Input: part model. Units: mm. Frame: model coordinates. A direction names the side the tool comes from. Round coordinates to 2 decimals unless told otherwise and drop trailing zeros. Loops run counter-clockwise (first coordinate to the right, second up) from the corner with the lowest first, then second, coordinate; pieces in that order, holes last. Notation, with made-up numbers: (70, -6.75) -> (112, -6.75) arc R11 ccw to (112, 1.25) -> close; hole circle Ø2 at (8.25, -25.75). An arc over 180 degrees is marked (long way). Answer in a Markdown table with one row per item. Add a question column.
Q1. Mould query, pull axis X, two halves, no side actions, for faces 5 (the face through (5, 40, -17)), 6 (the face through (-30, 40, -19)), 7 (the face through (11, 40, -19)), 8 (the face through (-10, 40, 0)). Classes: pulls with the +X half, pulls with the -X half, needs draft (parallel to the pull), parting line crosses it, or undercut.
Q2. Pin query (flat end, axial travel): pin 1 (5.5 mm diameter, centred on x = -6.5, y = 35.5, fed in from -Z); pin 2 (5 mm diameter, centred on x = 7, y = 40, fed in from +Z); pin 3 (10 mm diameter, centred on y = 44.5, z = -2.5, fed in from +X). Return the tip coordinate at first contact, or that it passes through.
Q3. Reachability of faces 1 (the face through (-10, 40, 3)), 2 (the face through (-22, 40, -7)), 3 (the face through (3, 40, -7)), 4 (the face through (-19, 40, -10)) from +Z, -Z, +X, -X, +Y, -Y: full face, straight path, thin tool, end or side. Return the list, or none.
Q4. Section A-A, the plane x = -26. Output: boundary loops of the cut face in (y, z), and give its area (3 significant figures).
Q5. Ray query, L1, parallel to X at y = 40, z = -18.55; L2, parallel to Y at x = -26, z = -18; L3, parallel to X at y = 33.5, z = -18.25. Return the intervals inside material, ascending. Write a range as from..to.
Q6. Section D-D, the plane y = 35.5. Output: boundary loops of the cut face in (x, z).
Q7. Section C-C, the plane z = -2.25. Output: boundary loops of the cut face in (x, y).
Q8. Section B-B, the plane y = 40. Output: boundary loops of the cut face in (x, z).
Autodesk Fusion 360 part; units mm, degrees
sketch "Sketch1" plane through (0, 0, 0) normal (1, 0, 0) x (0, 1, 0) in component "Integrated frame"
  circle A0 centre (-46.8244, 18.5) radius 1.5
  circle A1 centre (-9.8244, 18.5) radius 1.5
  circle A2 centre (-46.8244, -18.5) radius 1.5
  circle A3 centre (-9.8244, -18.5) radius 1.5
  line L0 (0, 0) -> (0, 35.4619) construction
  line L1 (60, 100) -> (-60, 100)
  line L2 (-60, 100) -> (-60, -100)
  line L3 (-60, -100) -> (60, -100)
  line L4 (60, -100) -> (60, 100)
  line L5 (60, 100) -> (-60, -100) construction
  line L6 (-60, 100) -> (60, -100) construction
  circle A4 centre (46.8244, 18.5) radius 1.5
  circle A5 centre (46.8244, -18.5) radius 1.5
  circle A6 centre (9.8244, -18.5) radius 1.5
  circle A7 centre (9.8244, 18.5) radius 1.5
  line L7 (-18.5, -45.3481) -> (-21.5, -45.3481)
  line L8 (-21.5, -45.3481) -> (-21.5, -70.3481)
  line L9 (-21.5, -70.3481) -> (-18.5, -70.3481)
  line L10 (-18.5, -70.3481) -> (-18.5, -45.3481)
  line L11 (21.5, -45.3481) -> (21.5, -70.3481)
  line L12 (18.5, -70.3481) -> (18.5, -45.3481)
  line L13 (18.5, -45.3481) -> (21.5, -45.3481)
  line L14 (21.5, -70.3481) -> (18.5, -70.3481)
  circle A8 centre (-43.3091, 82.7998) radius 1.5
  circle A9 centre (-21.3091, 82.7998) radius 1.5
  circle A10 centre (21.3091, 82.7998) radius 1.5
  circle A11 centre (43.3091, 82.7998) radius 1.5
  line L15 (0, 0) -> (33.4715, 0) construction
  circle A12 centre (-43.3091, -82.7998) radius 1.5
  circle A13 centre (-21.3091, -82.7998) radius 1.5
  circle A14 centre (43.3091, -82.7998) radius 1.5
  circle A15 centre (21.3091, -82.7998) radius 1.5
  point P0 (-28.3244, 0)
  dimension "d246" = 3
  dimension "d248" = 18.5
  dimension "d249" = 18.5
  dimension "d252" = 37
  dimension "d253" = -37
  dimension "d261" = 120
  dimension "d262" = 200
  dimension "d264" = 3
  dimension "d265" = 25
  dimension "d266" = 18.5
  dimension "d269" = 3
  dimension "d270" = 3
  dimension "d271" = 22
sketch "Sketch1 (2)" plane through (0, 0, 0) normal (0, 0, 1) x (1, 0, 0) in component "MotorClamp"
  line L0 (0, 50) -> (-19, 50)
  line L1 (-19, 50) -> (-19, 30)
  line L2 (-19, 30) -> (0, 30)
  line L3 (0, 30) -> (0, 50)
  line L4 (-19, 50) -> (-22, 50)
  line L5 (-22, 50) -> (-22, 30)
  line L6 (-22, 30) -> (-19, 30)
  line L7 (-19, 30) -> (-19, 50)
  line L8 (0, 50) -> (3, 50)
  line L9 (3, 50) -> (3, 30)
  line L10 (3, 30) -> (0, 30)
  line L11 (0, 30) -> (0, 50)
  dimension "d272" = 19
  dimension "d273" = 20
  dimension "d274" = 3
  dimension "d275" = 3
extrude "Extrude1" add sketch "Sketch1 (2)" along normal blind 3 in component "MotorClamp"
extrude "Extrude2" add sketch "Sketch1 (2)" against normal blind 17 contours L3 L8 L9 L10 L11 | L1 L4 L5 L6 L7 in component "MotorClamp"
extrude "Extrude3" add 2 faces at (-20, 36.6667, -17) (1, 43.3333, -17) along direction (0, 0, -1) blind 3 in component "MotorClamp"
sketch "Sketch2" plane through (0, 0, -20) normal (0, 0, -1) x (1, 0, 0) in component "MotorClamp"
  line L0 (-19, -50) -> (-19, -30)
  line L1 (-19, -30) -> (-22, -30)
  line L2 (-22, -30) -> (-22, -50)
  line L3 (-22, -50) -> (-19, -50)
  line L4 (-22, -30) -> (-30, -30)
  line L5 (-30, -30) -> (-30, -50)
  line L6 (-30, -50) -> (-22, -50)
  line L7 (-22, -50) -> (-22, -30)
  line L8 (3, -50) -> (11, -50)
  line L9 (11, -50) -> (11, -30)
  line L10 (11, -30) -> (3, -30)
  line L11 (3, -30) -> (3, -50)
  line L12 (-30, -30) -> (-22, -50) construction
  line L13 (-30, -50) -> (-22, -30) construction
  line L14 (3, -30) -> (11, -50) construction
  line L15 (3, -50) -> (11, -30) construction
  circle A0 centre (-26, -40) radius 1.55
  circle A1 centre (7, -40) radius 1.55
  dimension "d282" = 8
  dimension "d283" = 8
  dimension "d284" = 25
  dimension "d285" = 3.1
  dimension "d286" = 3.1
extrude "Extrude4" add sketch "Sketch2" against normal blind 3 contours L2 L4 L5 L6 L7 | L8 L9 L10 L11 in component "MotorClamp"
extrude "Extrude1'" [suppressed] in component "Integrated frame"
sketch "Laser cut sketch" plane through (3, 0, 0) normal (1, 0, 0) x (0, 1, 0) in component "Integrated frame"
  circle A0 centre (-9.8244, -18.5) radius 1.5
  circle A1 centre (-46.8244, -18.5) radius 1.5
  circle A2 centre (-46.8244, 18.5) radius 1.5
  circle A3 centre (-9.8244, 18.5) radius 1.5
  circle A4 centre (46.8244, 18.5) radius 1.5
  circle A5 centre (46.8244, -18.5) radius 1.5
  circle A6 centre (9.8244, -18.5) radius 1.5
  circle A7 centre (9.8244, 18.5) radius 1.5
  line L0 (-18.5, -45.3481) -> (-18.5, -70.3481)
  line L1 (-18.5, -70.3481) -> (-21.5, -70.3481)
  line L2 (-21.5, -70.3481) -> (-21.5, -45.3481)
  line L3 (-21.5, -45.3481) -> (-18.5, -45.3481)
  line L4 (21.5, -45.3481) -> (21.5, -70.3481)
  line L5 (21.5, -70.3481) -> (18.5, -70.3481)
  line L6 (18.5, -70.3481) -> (18.5, -45.3481)
  line L7 (18.5, -45.3481) -> (21.5, -45.3481)
  line L8 (60, -100) -> (60, 100)
  line L9 (60, 100) -> (-60, 100)
  line L10 (-60, 100) -> (-60, -100)
  line L11 (-60, -100) -> (60, -100)
extrude "Extrude2'" [suppressed]
component "Integrated frame" placed x (1, 0, 0) y (0, 1, 0) z (0, 0, 1) at (0, 0, 0)
component "MotorClamp" placed x (1, 0, 0) y (0, 1, 0) z (0, 0, 1) at (0, 0, 0)
equation "partLength = 250 mm"
equation "partWidth = 25 mm"
equation "boltHole = 3 mm"
equation "boltFromEdgesClose = 10 mm"
equation "boltGap = 12 mm"
equation "boltFromEdgesFar = 40 mm"
equation "boltGapFromSide = ( partWidth - boltGap ) / 2"
equation "boltGapDiag = boltGap * sqrt(2)"
equation "d246 = boltHole"
equation "d248 = ( 37 / 2 ) * 1 mm"
equation "d249 = ( 37 / 2 ) * 1 mm"
equation "d266 = ( 37 / 2 ) * 1 mm"
equation "d269 = boltHole"
equation "d270 = boltHole"
equation "d285 = boltHole + 0.1 mm"
equation "d286 = boltHole + 0.1 mm"
Answer block:
| question | item | result |
|---|---|---|
| 1 | face 5 | needs draft |
| 1 | face 6 | pulls with the -X half |
| 1 | face 7 | pulls with the +X half |
| 1 | face 8 | undercut |
| 2 | pin 1 | z = 0 |
| 2 | pin 2 | z = -17 |
| 2 | pin 3 | x = 3 |
| 3 | face 1 | +Z, +X, -X, +Y, -Y |
| 3 | face 2 | +Z, -X, +Y, -Y |
| 3 | face 3 | +Z, +X, +Y, -Y |
| 3 | face 4 | -Z, +Y, -Y |
| 4 | outline | (30, -20) -> (38.45, -20) -> (38.45, -17) -> (30, -17) -> close; (41.55, -20) -> (50, -20) -> (50, -17) -> (41.55, -17) -> close |
| 4 | area | 50.7 mm^2 |
| 5 | L1 | -30..-27.55, -24.45..-19, 0..5.45, 8.55..11 |
| 5 | L2 | 30..38.45, 41.55..50 |
| 5 | L3 | -30..-19, 0..11 |
| 6 | outline | (-30, -20) -> (-19, -20) -> (-19, 0) -> (0, 0) -> (0, -20) -> (11, -20) -> (11, -17) -> (3, -17) -> (3, 3) -> (-22, 3) -> (-22, -17) -> (-30, -17) -> close |
| 7 | outline | (-22, 30) -> (-19, 30) -> (-19, 50) -> (-22, 50) -> close; (0, 30) -> (3, 30) -> (3, 50) -> (0, 50) -> close |
| 8 | outline | (-30, -20) -> (-27.55, -20) -> (-27.55, -17) -> (-30, -17) -> close; (-24.45, -20) -> (-19, -20) -> (-19, 0) -> (0, 0) -> (0, -20) -> (5.45, -20) -> (5.45, -17) -> (3, -17) -> (3, 3) -> (-22, 3) -> (-22, -17) -> (-24.45, -17) -> close; (8.55, -20) -> (11, -20) -> (11, -17) -> (8.55, -17) -> close |
